The model under review builds one solid part; all positions refer to its coordinate system, in mm. A direction names the side the tool comes from. Round coordinates to 2 decimals unless told otherwise and drop trailing zeros. Write each loop counter-clockwise with the first axis right and the second up, starting at its lowest first coordinate (ties: lowest second). Pieces come first, ordered by that corner, then holes. Notation, with made-up numbers: (42, -3) -> (63, -3) arc R14 cw to (63, 7) -> close; hole circle Ø8 at (87.5, -22). An arc over 180 degrees is marked (long way). Return JSON: item names as keys, results as strings. Group by question number.
1. Take a section at A-A, the plane y = 3. Write out the cut boundary in (x, z) (1 decimal), then the cut area to 3 significant figures.
2. Mouldability with a two-part tool opening along X and no side actions: class faces 1 (the flat face through (-46, 13.589, 0)), 2 (the cylindrical face through (46.272, -1.424, 0.4)), 3 (the flat face through (-1, 0, 0)), 4 (the flat face through (-44.894, 7, 0)) as pulls with the +X half, pulls with the -X half, needs draft (parallel to the pull), parting line crosses it, or undercut.
3. Take a section at C-C, the plane x = 32. Write out the cut boundary in (y, z) (3 decimals), then the cut area to 3 significant figures.
4. Take a section at B-B, the plane z = 0.5. Write out the cut boundary in (x, y).
5. For line 1 along X through (y, z) = (9, 17); line 2 along Y through (x, z) = (-11.5, 19); line 3 along X through (y, z) = (52.5, 12.5), list the stretches that pass through material, from the lowest coordinate up. Write a range as from..to.
6. Tool access review of faces 5 (the flat face through (44.894, 35, 0)), 6 (the flat face through (46, 67.564, 0)): name each direction out of +Z, -Z, +X, -X, +Y, -Y from which nothing blocks a thin tool from reaching the whole face with its end or side.
7. Take a section at D-D, the plane y = 39.5. Write out the cut boundary in (x, z) (1 decimal), then the cut area to 3 significant figures.
8. Clearance check with flat-ended pins moving along their axes: P1, Ø17, axis at x = -14.5, z = -10.5, coming from the +Y side; P2, Ø5, axis at y = 48.5, z = 12.5, coming from the -X side; P3, Ø1.1, axis at x = -45.5, z = 3, coming from the +Y side. State where each tip first meets the part, or that it passes through.
from build123d import *

# Parameters (mm, degrees)
SKETCH1_W                    = 94.361
SKETCH1_H                    = 57.15
BASE_FLANGE1_DEPTH           = 2.286
EDGE_FLANGE1_STRIP_W         = 10.6172
EDGE_FLANGE1_STRIP_H         = 2.286
EDGE_FLANGE1_STRIP_CUT_DEPTH = 57.15
EDGE_FLANGE1_DEPTH           = 57.15
EDGE_FLANGE2_STRIP_W         = 10.6172
EDGE_FLANGE2_STRIP_H         = 2.286
EDGE_FLANGE2_STRIP_CUT_DEPTH = 57.15
EDGE_FLANGE2_DEPTH           = 57.15


# Sheet-metal steps are written as plain solids
with BuildPart() as part:
    # Sketch1 → Base-Flange1 (new body)
    with BuildSketch(Plane(origin=(0, 0, 0), x_dir=(1, 0, 0), z_dir=(0, 1, 0))):
        Rectangle(SKETCH1_W, SKETCH1_H)
    extrude(amount=-BASE_FLANGE1_DEPTH)

    # Edge-Flange1 strip (across the edge) → Edge-Flange1 strip cut (cut)
    with BuildSketch(Plane(origin=(-47.1805, 0, -28.575), x_dir=(1, 0, 0), z_dir=(0, 0, 1))):
        with Locations((-2.286, -1.143)):
            Rectangle(EDGE_FLANGE1_STRIP_W, EDGE_FLANGE1_STRIP_H)
    extrude(amount=EDGE_FLANGE1_STRIP_CUT_DEPTH, mode=Mode.SUBTRACT)

    # Edge-Flange1 section (across the edge) → Edge-Flange1 (add)
    with BuildSketch(Plane(origin=(-47.1805, 0, -28.575), x_dir=(1, 0, 0), z_dir=(0, 0, 1))):
        with BuildLine():
            Line((0, 0.7366), (0, 13.589))
            Line((0, 13.589), (2.286, 13.589))
            Line((2.286, 13.589), (2.286, 0.7366))
            ThreePointArc((2.286, 0.7366), (2.501745145, 0.215745145), (3.0226, 0))
            Line((3.0226, 0), (3.0226, -2.286))
            ThreePointArc((3.0226, -2.286), (0.885299043, -1.400700957), (0, 0.7366))
        make_face()
    extrude(amount=EDGE_FLANGE1_DEPTH)

    # Edge-Flange2 strip (across the edge) → Edge-Flange2 strip cut (cut)
    with BuildSketch(Plane(origin=(47.1805, 0, 28.575), x_dir=(-1, 0, 0), z_dir=(0, 0, -1))):
        with Locations((-2.286, -1.143)):
            Rectangle(EDGE_FLANGE2_STRIP_W, EDGE_FLANGE2_STRIP_H)
    extrude(amount=EDGE_FLANGE2_STRIP_CUT_DEPTH, mode=Mode.SUBTRACT)

    # Edge-Flange2 section (across the edge) → Edge-Flange2 (add)
    with BuildSketch(Plane(origin=(47.1805, 0, 28.575), x_dir=(-1, 0, 0), z_dir=(0, 0, -1))):
        with BuildLine():
            Line((0, 0.7366), (0, 67.564))
            Line((0, 67.564), (2.286, 67.564))
            Line((2.286, 67.564), (2.286, 0.7366))
            ThreePointArc((2.286, 0.7366), (2.501745145, 0.215745145), (3.0226, 0))
            Line((3.0226, 0), (3.0226, -2.286))
            ThreePointArc((3.0226, -2.286), (0.885299043, -1.400700957), (0, 0.7366))
        make_face()
    extrude(amount=EDGE_FLANGE2_DEPTH)


solid = part.part
Output:
{
 "1": {"outline": "(-47.2, -28.6) -> (-44.9, -28.6) -> (-44.9, 28.6) -> (-47.2, 28.6) -> close; (44.9, -28.6) -> (47.2, -28.6) -> (47.2, 28.6) -> (44.9, 28.6) -> close", "area": "261 mm^2"},
 "2": {"face 1": "needs draft", "face 2": "pulls with the +X half", "face 3": "undercut", "face 4": "undercut"},
 "3": {"outline": "(-2.286, -28.575) -> (0, -28.575) -> (0, 28.575) -> (-2.286, 28.575) -> close", "area": "131 mm^2"},
 "4": {"outline": "(-47.18, 0.74) arc R3.02 ccw to (-44.16, -2.29) -> (44.16, -2.29) arc R3.02 ccw to (47.18, 0.74) -> (47.18, 67.56) -> (44.89, 67.56) -> (44.89, 0.74) arc R0.74 cw to (44.16, 0) -> (-44.16, 0) arc R0.74 cw to (-44.89, 0.74) -> (-44.89, 13.59) -> (-47.18, 13.59) -> close"},
 "5": {"line 1": "x = -47.18..-44.89, 44.89..47.18", "line 2": "y = -2.29..0", "line 3": "x = 44.89..47.18"},
 "6": {"face 5": "+Z, -Z, +Y", "face 6": "+Z, -Z, +X, -X, +Y"},
 "7": {"outline": "(44.9, -28.6) -> (47.2, -28.6) -> (47.2, 28.6) -> (44.9, 28.6) -> close", "area": "131 mm^2"},
 "8": {"P1": "stops at y = 0", "P2": "stops at x = 44.89", "P3": "stops at y = 13.59"}
}
